from build123d import *

# Parameters (mm, degrees)
SKETCH156_R       = 3.2
EXTRUDE057_DEPTH  = 50
EXTRUDE054_DEPTH  = 10
CYLINDER179_R     = 2.8
CYLINDER179_DEPTH = 300
CYLINDER180_R     = 2.8
CYLINDER180_DEPTH = 300
EXTRUDE055_DEPTH  = 30
SKETCH152_R       = 93
SKETCH152_R_2     = 11
SKETCH152_R_3     = 15.1
SKETCH152_R_4     = 6.4
EXTRUDE053_DEPTH  = 8
EXTRUDE056_DEPTH  = 100
FILLET024_R       = 5
FILLET025_R       = 2
FILLET026_R       = 5
FILLET027_R       = 2.5


with BuildPart() as extrude057:
    # Sketch156 → Extrude057 (new body)
    with BuildSketch(Plane.XY):
        with Locations((0, -150)):
            Circle(SKETCH156_R)
        with Locations((0, -100)):
            Circle(SKETCH156_R)
    extrude(amount=EXTRUDE057_DEPTH)


with BuildPart() as extrude057_1:
    # Extrude057 placement: moved
    add(extrude057.part.moved(Location((0, 0, -290))))


with BuildPart() as obj1:
    # Sketch153 → Extrude054 (new body)
    with BuildSketch(Plane.XY):
        with BuildLine():
            ThreePointArc((-5, -220), (0, -225), (5, -220))
            Line((5, -220), (5, -212.5))
            ThreePointArc((5, -212.5), (0, -207.5), (-5, -212.5))
            Line((-5, -212.5), (-5, -220))
        make_face()
    extrude(amount=EXTRUDE054_DEPTH)


with BuildPart() as obj1_1:
    # Extrude054 placement: moved
    add(obj1.part.moved(Location((0, 0, -246.5))))


with BuildPart() as cylinder179:
    # Cylinder179 → Cylinder179 (new body)
    with BuildSketch(Plane(origin=(0, 0, 90), x_dir=(1, 0, 0), z_dir=(0, -1, 0))):
        Circle(CYLINDER179_R)
    extrude(amount=CYLINDER179_DEPTH)


with BuildPart() as m4heatsetcuts004:
    # Cylinder180 → Cylinder180 (new body)
    with BuildSketch(Plane(origin=(-150, -150, 90), x_dir=(0, 1, 0), z_dir=(1, 0, 0))):
        Circle(CYLINDER180_R)
    extrude(amount=CYLINDER180_DEPTH)

    # Fusion131: union Cylinder179
    add(cylinder179.part)


with BuildPart() as m4heatsetcuts004_1:
    # Fusion131 placement: moved
    add(m4heatsetcuts004.part.moved(Location((0, 0, -321))))


with BuildPart() as obj2:
    # Sketch154 → Extrude055 (new body)
    with BuildSketch(Plane.XY):
        with BuildLine():
            ThreePointArc((-89.576783, -125), (-93, -150), (-89.576783, -175))
            Line((-89.576783, -175), (-82.286086, -175))
            ThreePointArc((-82.286086, -125), (-86, -150), (-82.286086, -175))
            Line((-89.576783, -125), (-82.286086, -125))
        make_face()
        with BuildLine():
            ThreePointArc((25, -60.423217), (0, -57), (-25, -60.423217))
            Line((-25, -60.423217), (-25, -67.713914))
            ThreePointArc((25, -67.713914), (0, -64), (-25, -67.713914))
            Line((25, -60.423217), (25, -67.713914))
        make_face()
        with BuildLine():
            ThreePointArc((89.576783, -175), (93, -150), (89.576783, -125))
            Line((89.576783, -125), (82.286086, -125))
            ThreePointArc((82.286086, -175), (86, -150), (82.286086, -125))
            Line((89.576783, -175), (82.286086, -175))
        make_face()
        with BuildLine():
            ThreePointArc((-25, -239.576783), (0, -243), (25, -239.576783))
            Line((25, -239.576783), (25, -232.286086))
            ThreePointArc((-25, -232.286086), (0, -236), (25, -232.286086))
            Line((-25, -239.576783), (-25, -232.286086))
        make_face()
    extrude(amount=EXTRUDE055_DEPTH)


with BuildPart() as obj2_1:
    # Extrude055 placement: moved
    add(obj2.part.moved(Location((0, 0, -250))))


with BuildPart() as level5s009:
    # Sketch152 → Extrude053 (new body)
    with BuildSketch(Plane.XY):
        with Locations((0, -150)):
            Circle(SKETCH152_R)
        with Locations((-57, -150)):
            Circle(SKETCH152_R_2, mode=Mode.SUBTRACT)
        with Locations((57, -150)):
            Circle(SKETCH152_R_3, mode=Mode.SUBTRACT)
        with Locations((35, -200)):
            Circle(SKETCH152_R_3, mode=Mode.SUBTRACT)
        with Locations((-35, -200)):
            Circle(SKETCH152_R_4, mode=Mode.SUBTRACT)
        with BuildLine():
            ThreePointArc((-3.2, -216.158125), (0, -225), (3.2, -216.158125))
            Line((3.2, -216.158125), (3.2, -212.5))
            ThreePointArc((3.2, -212.5), (0, -209.3), (-3.2, -212.5))
            Line((-3.2, -212.5), (-3.2, -216.158125))
        make_face(mode=Mode.SUBTRACT)
    extrude(amount=EXTRUDE053_DEPTH)


with BuildPart() as level5s009_1:
    # Extrude053 placement: moved
    add(level5s009.part.moved(Location((0, 0, -250))))

    # Fusion130: union obj2
    add(obj2_1.part)

    # Cut095: cut m4HeatSetCuts004
    add(m4heatsetcuts004_1.part, mode=Mode.SUBTRACT)

    # Cut096: cut obj1
    add(obj1_1.part, mode=Mode.SUBTRACT)


with BuildPart() as obj3:
    # Sketch155 → Extrude056 (new body)
    with BuildSketch(Plane.XZ):
        Polygon((-20.75, -250), (-12.75, -250), (-12.75, -275.75), (12.75, -275.75), (12.75, -250), (20.75, -250), (20.75, -283.75), (-20.75, -283.75), align=None)
    extrude(amount=EXTRUDE056_DEPTH)


with BuildPart() as obj3_1:
    # Extrude056 placement: moved
    add(obj3.part.moved(Location((0, -70, 0))))

    # Fillet024
    fillet024_edges = [obj3_1.edges().sort_by_distance(p)[0] for p in [
        (20.75, -120, -283.75),
        (-20.75, -120, -283.75),
    ]]
    fillet(fillet024_edges, radius=FILLET024_R)

    # Fillet025
    fillet025_edges = [obj3_1.edges().sort_by_distance(p)[0] for p in [
        (12.75, -120, -275.75),
        (-12.75, -120, -275.75),
    ]]
    fillet(fillet025_edges, radius=FILLET025_R)

    # Fusion132: union level5s009
    add(level5s009_1.part)

    # Fillet026
    fillet026_edges = [obj3_1.edges().sort_by_distance(p)[0] for p in [
        (-20.75, -120, -250),
        (20.75, -120, -250),
    ]]
    fillet(fillet026_edges, radius=FILLET026_R)

    # Cut097: cut Extrude057
    add(extrude057_1.part, mode=Mode.SUBTRACT)

    # Fillet027
    fillet027_edges = [obj3_1.edges().sort_by_distance(p)[0] for p in [
        (86, -150, -242),
        (0, -64, -242),
        (0, -236, -242),
        (-86, -150, -242),
    ]]
    fillet(fillet027_edges, radius=FILLET027_R)


solid = obj3_1.part
Could you check a few things on this model? Use its own coordinates, in mm. A direction names the side the tool comes from. Give positions to 0.01 mm unless a question says otherwise; leave off trailing zeros. Order: outer loops, then holes, each group sorted by start corner. A loop starts at its lowest first (then second) coordinate and runs counter-clockwise, first axis right, second up.
1. Suppose I cut it at D-D (y = -100). List the corners of the cut face in (x, z) for me, plus the area to 3 significant figures.
2. We'd pull the mould along Z, two halves only. Please class faces 1 (the flat face through (-12.75, -119, -262)), 2 (the cylindrical face through (19.32, -120.7, -282.25)), 3 (the cylindrical face through (-58.432, -139.094, -246.056)): pulls with the +Z half, pulls with the -Z half, needs draft (parallel to the pull), parting line crosses it, or undercut.
3. Will these pins go through, and if not, where does the flat tip stop? P1, Ø1.5, axis at y = -159, z = -250.5, coming from the +X side; P2, Ø5, axis at x = -1, y = -213, coming from the +Z side; P3, Ø5, axis at x = -85.5, z = -233.5, coming from the -Y side.
4. I need wall thicknesses on L1, parallel to Y at x = 0, z = -245.5; L2, parallel to Y at x = 0, z = -248; L3, parallel to Z at x = -2.5, y = -122.5. Which ranges of each line are inside material? Lowest first, please.
5. Suppose I cut it at A-A (z = -223.5). List the corners of the cut face in (x, y) for me.
6. For faces 4 (the flat face through (-20.75, -119, -267)), 5 (the flat face through (-86, -125, -231)), 6 (the flat face through (5, -216, -244)), 7 (the flat face through (25, -236, -231)), which set-ups out of +Z, -Z, +X, -X, +Y, -Y let a thin tool reach every point of the face, with its end or its side?
7. Suppose I cut it at C-C (z = -271.5). List the corners of the cut face in (x, y) for me.
8. Suppose I cut it at B-B (x = 68.5). List the corners of the cut face in (y, z) for me.
Solved:
1. outline: (-78.42, -250) - (-25.75, -250) arc R5 cw to (-20.75, -255) - (-20.75, -278.75) arc R5 ccw to (-15.75, -283.75) - (-3.2, -283.75) - (-3.2, -275.75) - (-10.75, -275.75) arc R2 cw to (-12.75, -273.75) - (-12.75, -250) - (-3.2, -250) - (-3.2, -242) - (-78.42, -242) - close; (3.2, -283.75) - (15.75, -283.75) arc R5 ccw to (20.75, -278.75) - (20.75, -255) arc R5 cw to (25.75, -250) - (78.42, -250) - (78.42, -242) - (3.2, -242) - (3.2, -250) - (12.75, -250) - (12.75, -273.75) arc R2 cw to (10.75, -275.75) - (3.2, -275.75) - close
1. area: 1,900 mm2
2. face 1: undercut
2. face 2: pulls with the -Z half
2. face 3: needs draft
3. P1: stops at x = 92.62
3. P2: stops at z = -246.5
3. P3: stops at y = -175
4. L1: y = -243 to -225, -207.5 to -153.2, -146.8 to -103.2, -96.8 to -57
4. L2: y = -243 to -225, -209.3 to -153.2, -146.8 to -103.2, -96.8 to -57
4. L3: z = -283.75 to -275.75, -250 to -242
5. outline: (-89.58, -175) - (-82.29, -175) arc R86 cw to (-82.29, -125) - (-89.58, -125) arc R93 ccw to start; (-25, -239.58) arc R93 ccw to (25, -239.58) - (25, -232.29) arc R86 cw to (-25, -232.29) - close; (-25, -67.71) arc R86 cw to (25, -67.71) - (25, -60.42) arc R93 ccw to (-25, -60.42) - close; (82.29, -175) - (89.58, -175) arc R93 ccw to (89.58, -125) - (82.29, -125) arc R86 cw to start
6. face 4: -Z, -X, +Y, -Y
6. face 5: +Z, +X, -X, +Y
6. face 6: +Z
6. face 7: +Z, +X, +Y, -Y
7. outline: (-20.75, -170) - (-12.75, -170) - (-12.75, -70) - (-20.75, -70) - close; (12.75, -170) - (20.75, -170) - (20.75, -70) - (12.75, -70) - close
8. outline: (-212.9, -250) - (-159.79, -250) - (-159.79, -242) - (-212.9, -242) - close; (-140.21, -250) - (-87.1, -250) - (-87.1, -242) - (-140.21, -242) - close
